from build123d import *

# Parameters (mm, degrees)
SKETCH1_W                = 41.91
SKETCH1_H                = 9.652
BOSS_EXTRUDE1_DEPTH      = 26.67
SKETCH2_R                = 1.651
CUT_EXTRUDE1_DEPTH       = 51.605316954
SKETCH3_R                = 2.159
CUT_EXTRUDE2_DEPTH       = 6.35
CHAMFER5_SIZE            = 0.762
SKETCH5_R                = 2.159
CUT_EXTRUDE4_DEPTH       = 5.08
SKETCH6_R                = 2.921
CUT_EXTRUDE5_DEPTH       = 0.762
CHAMFER2_SIZE            = 0.762
SKETCH7_R                = 0.762
CUT_EXTRUDE6_DEPTH       = 5.334
SKETCH9_R                = 1.016
CUT_EXTRUDE7_DEPTH       = 1.27
SKETCH10_R               = 1.397
CUT_EXTRUDE8_DEPTH       = 0.762
CHAMFER3_SIZE            = 0.508
CHAMFER3_OF_MIRROR2_SIZE = 0.508
SKETCH12_R               = 0.762
CUT_EXTRUDE9_DEPTH       = 4.572
SKETCH14_R               = 1.016
CUT_EXTRUDE10_DEPTH      = 0.254
CHAMFER4_SIZE            = 0.254
CHAMFER4_OF_MIRROR3_SIZE = 0.254


# Some blends are built 0.0001 mm under size
with BuildPart() as part:
    # Sketch1 → Boss-Extrude1 (new body)
    with BuildSketch(Plane(origin=(0, 0, 0), x_dir=(1, 0, 0), z_dir=(0, 1, 0))):
        with Locations((20.955, 4.826)):
            Rectangle(SKETCH1_W, SKETCH1_H)
    extrude(amount=BOSS_EXTRUDE1_DEPTH)

    # Sketch2 → Cut-Extrude1 (cut, through all)
    with BuildSketch(Plane.XY):
        with Locations((34.29, 22.606)):
            Circle(SKETCH2_R)
        with Locations(Location((7.62, 22.606, 0), (0, 0, 180))):
            Circle(SKETCH2_R)
    extrude(amount=-CUT_EXTRUDE1_DEPTH, mode=Mode.SUBTRACT)

    # Sketch3 → Cut-Extrude2 (cut)
    with BuildSketch(Plane(origin=(0, 26.67, 0), x_dir=(1, 0, 0), z_dir=(0, 1, 0))):
        with Locations(Location((25.273, 4.826, 0), (0, 0, 270))):
            Circle(SKETCH3_R)
        with Locations(Location((16.637, 4.826, 0), (0, 0, 90))):
            Circle(SKETCH3_R)
    extrude(amount=-CUT_EXTRUDE2_DEPTH, mode=Mode.SUBTRACT)

    # Chamfer5
    chamfer5_edges = [part.edges().sort_by_distance(p)[0] for p in [
        (25.273, 26.67, -6.985),
        (16.637, 26.67, -2.667),
    ]]
    chamfer(chamfer5_edges, length=CHAMFER5_SIZE)

    # Sketch5 → Cut-Extrude4 (cut)
    with BuildSketch(Plane(origin=(0, 0, 0), x_dir=(-1, 0, 0), z_dir=(0, -1, 0))):
        with Locations(Location((-33.401, 4.826, 0), (0, 0, 90))):
            Circle(SKETCH5_R)
        with Locations(Location((-8.509, 4.826, 0), (0, 0, 270))):
            Circle(SKETCH5_R)
        with Locations(Location((-20.955, 4.826, 0), (0, 0, 90))):
            Circle(SKETCH5_R)
    extrude(amount=-CUT_EXTRUDE4_DEPTH, mode=Mode.SUBTRACT)

    # Sketch6 → Cut-Extrude5 (cut)
    with BuildSketch(Plane(origin=(0, 0, 0), x_dir=(-1, 0, 0), z_dir=(0, -1, 0))):
        with Locations(Location((-33.401, 4.826, 0), (0, 0, 90))):
            Circle(SKETCH6_R)
        with Locations(Location((-20.955, 4.826, 0), (0, 0, 90))):
            Circle(SKETCH6_R)
        with Locations(Location((-8.509, 4.826, 0), (0, 0, 90))):
            Circle(SKETCH6_R)
    extrude(amount=-CUT_EXTRUDE5_DEPTH, mode=Mode.SUBTRACT)

    # Chamfer2
    chamfer2_edges = [part.edges().sort_by_distance(p)[0] for p in [
        (33.401, 0.762, -1.905),
        (20.955, 0.762, -1.905),
        (8.509, 0.762, -1.905),
    ]]
    chamfer(chamfer2_edges, length=CHAMFER2_SIZE - 0.0001)  # a hair under: the kernel refuses the full size

    # Sketch7 → Cut-Extrude6 (cut)
    with BuildSketch(Plane(origin=(41.91, 0, 0), x_dir=(0, 0, -1), z_dir=(1, 0, 0))):
        with Locations((2.286, 2.54)):
            Circle(SKETCH7_R)
    cut_extrude6 = extrude(amount=-CUT_EXTRUDE6_DEPTH, mode=Mode.SUBTRACT)

    # Sketch9 → Cut-Extrude7 (cut)
    with BuildSketch(Plane(origin=(41.91, 0, 0), x_dir=(0, 0, -1), z_dir=(1, 0, 0))):
        with Locations((2.286, 2.54)):
            Circle(SKETCH9_R)
    cut_extrude7 = extrude(amount=-CUT_EXTRUDE7_DEPTH, mode=Mode.SUBTRACT)

    # Sketch10 → Cut-Extrude8 (cut)
    with BuildSketch(Plane(origin=(41.91, 0, 0), x_dir=(0, 0, -1), z_dir=(1, 0, 0))):
        with Locations((2.286, 2.54)):
            Circle(SKETCH10_R)
    cut_extrude8 = extrude(amount=-CUT_EXTRUDE8_DEPTH, mode=Mode.SUBTRACT)

    # Chamfer3
    # the kernel refuses this chamfer: 0.508 mm, written as the material it adds along each edge
    with BuildSketch(Plane(origin=(40.64, 2.54, -2.286), x_dir=(0, 0, -1), z_dir=(0, -1, 0))) as chamfer3_piece_1_section:
        Polygon((1.016, CHAMFER3_SIZE), (1.016 - CHAMFER3_SIZE, 0), (1.016, 0), align=None)
    chamfer3_piece_1 = revolve(axis=Axis((40.64, 2.54, -2.286), (1, 0, 0)), mode=Mode.PRIVATE)
    chamfer3_piece_1 = split(chamfer3_piece_1, bisect_by=Plane(origin=(41.148, 2.54, -1.391029136), z_dir=(-1, 0, 0)), keep=Keep.TOP, mode=Mode.PRIVATE)
    chamfer3_piece_1 = chamfer3_piece_1 - Plane(origin=(41.015029136, 2.54, -2.286), x_dir=(0, 0, -1), z_dir=(1, 0, 0)) * Cylinder(0.762, 5, mode=Mode.PRIVATE)
    add(chamfer3_piece_1)

    # Mirror2: Cut-Extrude6, Cut-Extrude7, Cut-Extrude8 across plane
    add(cut_extrude6.mirror(Plane.ZY.offset(-20.955)), mode=Mode.SUBTRACT)
    add(cut_extrude7.mirror(Plane.ZY.offset(-20.955)), mode=Mode.SUBTRACT)
    add(cut_extrude8.mirror(Plane.ZY.offset(-20.955)), mode=Mode.SUBTRACT)

    # Chamfer3 of Mirror2
    # the kernel refuses this chamfer: 0.508 mm, written as the material it adds along each edge
    with BuildSketch(Plane(origin=(1.27, 2.54, -2.286), x_dir=(0, 0, -1), z_dir=(0, -1, 0))) as chamfer3_of_mirror2_piece_1_section:
        Polygon((1.016, -CHAMFER3_OF_MIRROR2_SIZE), (1.016 - CHAMFER3_OF_MIRROR2_SIZE, 0), (1.016, 0), align=None)
    chamfer3_of_mirror2_piece_1 = revolve(axis=Axis((1.27, 2.54, -2.286), (1, 0, 0)), mode=Mode.PRIVATE)
    chamfer3_of_mirror2_piece_1 = split(chamfer3_of_mirror2_piece_1, bisect_by=Plane(origin=(0.762, 2.54, -1.391029136), z_dir=(1, 0, 0)), keep=Keep.TOP, mode=Mode.PRIVATE)
    chamfer3_of_mirror2_piece_1 = chamfer3_of_mirror2_piece_1 - Plane(origin=(0.894970864, 2.54, -2.286), x_dir=(0, 0, -1), z_dir=(-1, 0, 0)) * Cylinder(0.762, 5, mode=Mode.PRIVATE)
    add(chamfer3_of_mirror2_piece_1)

    # Sketch12 → Cut-Extrude9 (cut)
    with BuildSketch(Plane.ZY):
        with Locations((-2.032, 22.098)):
            Circle(SKETCH12_R)
        with Locations(Location((-7.62, 22.098, 0), (0, 0, 180))):
            Circle(SKETCH12_R)
    cut_extrude9 = extrude(amount=-CUT_EXTRUDE9_DEPTH, mode=Mode.SUBTRACT)

    # Sketch14 → Cut-Extrude10 (cut)
    with BuildSketch(Plane.ZY):
        with Locations((-7.62, 22.098)):
            Circle(SKETCH14_R)
        with Locations((-2.032, 22.098)):
            Circle(SKETCH14_R)
    cut_extrude10 = extrude(amount=-CUT_EXTRUDE10_DEPTH, mode=Mode.SUBTRACT)

    # Chamfer4
    chamfer4_edges = [part.edges().sort_by_distance(p)[0] for p in [
        (0.254, 22.098, -8.636),
        (0.254, 22.098, -3.048),
    ]]
    chamfer(chamfer4_edges, length=CHAMFER4_SIZE - 0.0001)  # a hair under: the kernel refuses the full size

    # Mirror3: Cut-Extrude9, Cut-Extrude10 across plane
    add(cut_extrude9.mirror(Plane.ZY.offset(-20.955)), mode=Mode.SUBTRACT)
    add(cut_extrude10.mirror(Plane.ZY.offset(-20.955)), mode=Mode.SUBTRACT)

    # Chamfer4 of Mirror3
    chamfer4_of_mirror3_edges = [part.edges().sort_by_distance(p)[0] for p in [
        (41.656, 22.098, -8.636),
        (41.656, 22.098, -3.048),
    ]]
    chamfer(chamfer4_of_mirror3_edges, length=CHAMFER4_OF_MIRROR3_SIZE - 0.0001)  # a hair under: the kernel refuses the full size


solid = part.part
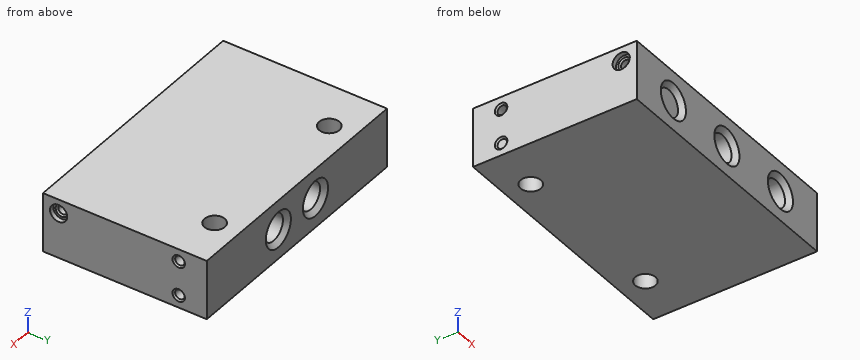
Source: CAD feature listing. Evaluate the final solid. Frame: model axes, mm. Round coordinates to 2 decimals unless told otherwise and drop trailing zeros. Write each loop counter-clockwise with the first axis right and the second up, starting at its lowest first coordinate (ties: lowest second). Pieces come first, ordered by that corner, then holes. Notation, with made-up numbers: (-8.75, 3) - (5.25, 3) arc R19 cw to (5.25, 23) - close; hole circle Ø2 at (-27.5, 61). An arc over 180 degrees is marked (long way). Use CSV: the item, a comma, the result in double quotes. Start each with the question number.
(1) Material intervals for probe 1 along X at (y, z) = (22.75, -1.25); probe 2 along Y at (x, z) = (3.5, -2.5); probe 3 along Y at (x, z) = (7.62, -4.5) (3 decimals), sorted ascending. Write a range as [from, to].
(2) Cut plane B-B, the plane y = 2.54. Return loops of the section in (x, z) (3 decimals).
(3) First-contact query: pin 1 Ø1.2 at (y, z) = (22.098, -2.032) entering from -X; pin 2 Ø0.8 at (y, z) = (22.5, -7.5) entering from +X; pin 3 Ø2.5 at (y, z) = (2.54, -2.286) entering from +X. Flat tips, straight axial feed; report the tip coordinate or a pass-through.
(4) Cut plane A-A, the plane x = 4. Return loops of the section in (y, z).
Geometry says:
1,probe 1,"[0, 5.98], [9.26, 32.65], [35.93, 41.91]"
1,probe 2,"[0, 1.81], [3.27, 21.5], [22.7, 26.67]"
1,probe 3,"[5.08, 20.955], [24.257, 26.67]"
2,outline,"(0, -9.652) - (41.91, -9.652) - (41.91, -3.683) - (41.148, -3.683) - (41.148, -3.302) - (40.894, -3.048) - (36.576, -3.048) - (36.576, -1.524) - (40.894, -1.524) - (41.148, -1.27) - (41.148, -0.889) - (41.91, -0.889) - (41.91, 0) - (0, 0) - (0, -0.889) - (0.762, -0.889) - (0.762, -1.27) - (1.016, -1.524) - (5.334, -1.524) - (5.334, -3.048) - (1.016, -3.048) - (0.762, -3.302) - (0.762, -3.683) - (0, -3.683) - close; hole circle Ø4.318 at (8.509, -4.826); hole circle Ø4.318 at (20.955, -4.826); hole circle Ø4.318 at (33.401, -4.826)"
3,pin 1,"x = 4.57"
3,pin 2,"x = 41.71"
3,pin 3,"x = 41.15"
4,outline,"(0, -9.65) - (26.67, -9.65) - (26.67, 0) - (0, 0) - close; hole circle Ø1.52 at (2.54, -2.29); hole circle Ø1.52 at (22.1, -7.62); hole circle Ø1.52 at (22.1, -2.03)"
